Model file for the job. Use its own axes, mm. Round coordinates to 2 decimals unless told otherwise and drop trailing zeros. Answer as CSV lines item,"result". Start each with the question number.
1. Pull direction Y, two halves, no side cores. Call faces 1 (the face through (48, 0, 2)), 2 (the face through (11.75, 2.53, 1.01)), 3 (the face through (-8.25, 2.53, 1.01)), 4 (the face through (-3, -7, 5)): released by +Y, released by -Y, zero draft, split by the parting line, or undercut.
2. Wall check: line 1 along Y through (x, z) = (25, 1.1); line 2 along Z through (x, y) = (9, 2); line 3 along Z through (x, y) = (40, 1.5). Give the ranges that are in metal, low to high. Write a range as [from, to].
3. Pin check, flat tips, straight feed: pin 1 Ø2 at (y, z) = (-5.5, 4.5) entering from -X; pin 2 Ø0.9 at (x, y) = (15, 0) entering from +Z; pin 3 Ø2 at (x, y) = (-29.97, 2.51) entering from +Z; pin 4 Ø1.6 at (x, z) = (22.5, 5.5) entering from +Y. Stop position of each tip, or through.
```python
from build123d import *

# Parameters (mm, degrees)
F0_R     = 2
F1_DEPTH = 4
F2_DEPTH = 5
F3_DEPTH = 7
F4_DEPTH = 2
F5_R     = 0.75
F5_R_2   = 0.7
F6_DEPTH = 25
F7_R     = 1


with BuildPart() as f1:
    # F0 (on Top) → F1 (new body)
    with BuildSketch(Plane.XY):
        with BuildLine():
            Line((-38.977494, -9.75), (0, -9.75))
            Line((0, -9.75), (38.977494, -9.75))
            ThreePointArc((38.977494, -9.75), (47.998028, -0.177918), (39.370675, 9.75))
            Line((39.370675, 9.75), (0, 9.75))
            Line((0, 9.75), (-39.370675, 9.75))
            ThreePointArc((-39.370675, 9.75), (-47.998028, -0.177918), (-38.977494, -9.75))
        make_face()
        with Locations((-43.5, 0)):
            Circle(F0_R, mode=Mode.SUBTRACT)
        with BuildLine():
            ThreePointArc((-32.335569, -7.688448), (-39.696451, -0.275465), (-32.78809, 7.560953))
            Line((-32.78809, 7.560953), (32.78809, 7.560953))
            ThreePointArc((32.78809, 7.560953), (39.696451, -0.275465), (32.335569, -7.688448))
            Line((32.335569, -7.688448), (32.202672, -7.692434))
            Line((32.202672, -7.692434), (-32.202672, -7.692434))
            Line((-32.202672, -7.692434), (-32.335569, -7.688448))
        make_face(mode=Mode.SUBTRACT)
        with Locations((43.5, 0)):
            Circle(F0_R, mode=Mode.SUBTRACT)
    extrude(amount=F1_DEPTH)

    # F0 (on Top) → F2 (join)
    with BuildSketch(Plane.XY):
        with BuildLine():
            Line((32.78809, 7.560953), (-32.78809, 7.560953))
            ThreePointArc((-32.78809, 7.560953), (-39.696451, -0.275465), (-32.335569, -7.688448))
            Line((-32.335569, -7.688448), (-32.202672, -7.692434))
            Line((-32.202672, -7.692434), (32.202672, -7.692434))
            Line((32.202672, -7.692434), (32.335569, -7.688448))
            ThreePointArc((32.335569, -7.688448), (39.696451, -0.275465), (32.78809, 7.560953))
        make_face()
        with BuildLine():
            Line((-31.980952, 6.095746), (-0.002622, 6.276632))
            Line((-0.002622, 6.276632), (31.953452, 6.276632))
            ThreePointArc((31.953452, 6.276632), (38.198581, 0.113907), (32.161089, -6.252371))
            Line((32.161089, -6.252371), (-32.165032, -6.192614))
            ThreePointArc((-32.165032, -6.192614), (-38.199125, 0.043335), (-31.980952, 6.095746))
        make_face(mode=Mode.SUBTRACT)
    extrude(amount=F2_DEPTH)

    # F0 (on Top) → F3 (join)
    with BuildSketch(Plane.XY):
        with BuildLine():
            Line((31.953452, 6.276632), (-0.002622, 6.276632))
            Line((-0.002622, 6.276632), (-31.980952, 6.095746))
            ThreePointArc((-31.980952, 6.095746), (-38.199125, 0.043335), (-32.165032, -6.192614))
            Line((-32.165032, -6.192614), (32.161089, -6.252371))
            ThreePointArc((32.161089, -6.252371), (38.198581, 0.113907), (31.953452, 6.276632))
        make_face()
        with BuildLine():
            ThreePointArc((-29.439345, -4.707238), (-34.69993, -0.04857), (-29.439345, 4.610098))
            Line((-29.439345, 4.610098), (30.636781, 4.776632))
            ThreePointArc((30.636781, 4.776632), (34.693866, 0.271074), (31.09103, -4.605355))
            Line((31.09103, -4.605355), (-29.439345, -4.707238))
        make_face(mode=Mode.SUBTRACT)
    extrude(amount=F3_DEPTH)

    # F0 (on Top) → F4 (join)
    with BuildSketch(Plane.XY):
        with BuildLine():
            Line((30.636781, 4.776632), (-29.439345, 4.610098))
            ThreePointArc((-29.439345, 4.610098), (-34.69993, -0.04857), (-29.439345, -4.707238))
            Line((-29.439345, -4.707238), (31.09103, -4.605355))
            ThreePointArc((31.09103, -4.605355), (34.693866, 0.271074), (30.636781, 4.776632))
        make_face()
    extrude(amount=F4_DEPTH)

    # F5 (on face) → F6 (cut)
    with BuildSketch(Plane.XY.offset(2)):
        with BuildLine():
            ThreePointArc((0, 0.75), (-0.75, 0), (0, -0.75))
            ThreePointArc((0, -0.75), (0.75, 0), (0, 0.75))
        make_face()
        with BuildLine():
            ThreePointArc((0, 3.25), (-0.75, 2.5), (0, 1.75))
            ThreePointArc((0, 1.75), (0.75, 2.5), (0, 3.25))
        make_face()
        with Locations((2.5, 0)):
            Circle(F5_R)
        with Locations((2.5, 2.5)):
            Circle(F5_R)
        with Locations((5, 0)):
            Circle(F5_R)
        with Locations((5, 2.5)):
            Circle(F5_R)
        with Locations((7.5, 0)):
            Circle(F5_R)
        with Locations((7.5, 2.5)):
            Circle(F5_R)
        with Locations((10, 0)):
            Circle(F5_R)
        with Locations((10, 2.5)):
            Circle(F5_R)
        with Locations((12.5, 0)):
            Circle(F5_R)
        with Locations((12.5, 2.5)):
            Circle(F5_R)
        with Locations((15, 0)):
            Circle(F5_R)
        with Locations((15, 2.5)):
            Circle(F5_R)
        with Locations((17.5, 0)):
            Circle(F5_R)
        with Locations((17.5, 2.5)):
            Circle(F5_R)
        with Locations((20, 0)):
            Circle(F5_R)
        with Locations((20, 2.5)):
            Circle(F5_R)
        with Locations((22.5, 0)):
            Circle(F5_R)
        with Locations((22.5, 2.5)):
            Circle(F5_R)
        with Locations((25, 0)):
            Circle(F5_R)
        with Locations((25, 2.5)):
            Circle(F5_R)
        with Locations((27.5, 0)):
            Circle(F5_R)
        with Locations((27.5, 2.5)):
            Circle(F5_R)
        with Locations((2.5, -2.5)):
            Circle(F5_R)
        with Locations((5, -2.5)):
            Circle(F5_R)
        with Locations((7.5, -2.5)):
            Circle(F5_R)
        with Locations((10, -2.5)):
            Circle(F5_R)
        with Locations((12.5, -2.5)):
            Circle(F5_R)
        with Locations((15, -2.5)):
            Circle(F5_R)
        with Locations((17.5, -2.5)):
            Circle(F5_R)
        with Locations((20, -2.5)):
            Circle(F5_R)
        with Locations((22.5, -2.5)):
            Circle(F5_R)
        with Locations((25, -2.5)):
            Circle(F5_R)
        with Locations((27.5, -2.5)):
            Circle(F5_R)
        with Locations((-12.5, 0)):
            Circle(F5_R)
        with Locations((-17.5, 0)):
            Circle(F5_R)
        with Locations((-7.5, 0)):
            Circle(F5_R)
        with Locations((-5, 0)):
            Circle(F5_R)
        with Locations((-15, 0)):
            Circle(F5_R)
        with Locations((-20, 0)):
            Circle(F5_R)
        with Locations((-10, 0)):
            Circle(F5_R)
        with Locations((-12.5, 2.5)):
            Circle(F5_R)
        with Locations((-10, 2.5)):
            Circle(F5_R)
        with Locations((-7.5, 2.5)):
            Circle(F5_R)
        with Locations((-5, 2.5)):
            Circle(F5_R)
        with Locations((-2.5, 0)):
            Circle(F5_R)
        with Locations((-2.5, 2.5)):
            Circle(F5_R)
        with Locations((-17.5, 2.5)):
            Circle(F5_R)
        with Locations((-15, 2.5)):
            Circle(F5_R)
        with Locations((-20, 2.5)):
            Circle(F5_R)
        with Locations((-27.5, 0)):
            Circle(F5_R)
        with Locations((-22.5, 0)):
            Circle(F5_R)
        with Locations((-25, 0)):
            Circle(F5_R)
        with Locations((-27.5, -2.5)):
            Circle(F5_R)
        with Locations((-25, 2.5)):
            Circle(F5_R)
        with Locations((-22.5, 2.5)):
            Circle(F5_R)
        with Locations((-17.5, -2.5)):
            Circle(F5_R)
        with Locations((-27.5, 2.5)):
            Circle(F5_R)
        with Locations((-20, -2.5)):
            Circle(F5_R)
        with Locations((-22.5, -2.5)):
            Circle(F5_R)
        with Locations((-25, -2.5)):
            Circle(F5_R)
        with Locations((-2.5, -2.5)):
            Circle(F5_R)
        with Locations((-5, -2.5)):
            Circle(F5_R)
        with Locations((-7.5, -2.5)):
            Circle(F5_R)
        with Locations((-10, -2.5)):
            Circle(F5_R)
        with Locations((-12.5, -2.5)):
            Circle(F5_R)
        with Locations((-15, -2.5)):
            Circle(F5_R)
        with Locations((0.020794, -2.485011)):
            Circle(F5_R_2)
        with Locations((-29.956931, 0.036661)):
            Circle(F5_R)
        with Locations((29.956931, 0.036661)):
            Circle(F5_R)
        with Locations((29.949998, 2.5)):
            Circle(F5_R)
        with Locations((32.449998, 2.5)):
            Circle(F5_R)
        with Locations((29.949998, -2.5)):
            Circle(F5_R)
        with Locations((32.449998, 0)):
            Circle(F5_R)
        with Locations((32.449998, -2.5)):
            Circle(F5_R)
        with Locations((-32.466013, 0.00955)):
            Circle(F5_R)
        with Locations((-32.466013, -2.49045)):
            Circle(F5_R)
        with Locations((-29.966013, 2.50955)):
            Circle(F5_R)
        with Locations((-32.466013, 2.50955)):
            Circle(F5_R)
        with Locations((-29.966013, -2.49045)):
            Circle(F5_R)
    extrude(amount=-F6_DEPTH, mode=Mode.SUBTRACT)

    # F7
    f7_edges = [f1.edges().sort_by_distance(p)[0] for p in [
        (-45.5, 0, 4),
        (41.5, 0, 4),
    ]]
    fillet(f7_edges, radius=F7_R)


solid = f1.part
```
Reply:
1,face 1,"split by the parting line"
1,face 2,"undercut"
1,face 3,"undercut"
1,face 4,"zero draft"
2,line 1,"y = [-9.75, -3.25], [-1.75, -0.75], [0.75, 1.75], [3.25, 9.75]"
2,line 2,"z = [0, 2]"
2,line 3,"z = [0, 4]"
3,pin 1,"stops at x = -46.82"
3,pin 2,"passes through"
3,pin 3,"stops at z = 2"
3,pin 4,"stops at y = 7.56"
